from build123d import *

# Parameters (mm, degrees)
EXTRUDE_1_DEPTH     = 6
SKETCH_2_R          = 12
EXTRUDE_2_DEPTH     = 3
SKETCH_3_R          = 4.1
CUT_EXTRUDE_1_DEPTH = 64.788713735
CUT_EXTRUDE_2_DEPTH = 2
FILLET_1_R          = 0.5
SKETCH_5_R          = 12
SKETCH_5_R_2        = 4.1
EXTRUDE_3_DEPTH     = 6
FILLET_2_R          = 2


with BuildPart() as part:
    # Sketch 1 → Extrude 1 (new body)
    with BuildSketch(Plane(origin=(0, 0, 0), x_dir=(1, 0, 0), z_dir=(0, 1, 0))):
        with BuildLine():
            Line((-50, 9), (50, 9))
            ThreePointArc((50, 9), (59, 0), (50, -9))
            Line((50, -9), (-50, -9))
            ThreePointArc((-50, -9), (-59, 0), (-50, 9))
        make_face()
    extrude(amount=EXTRUDE_1_DEPTH)

    # Sketch 2 → Extrude 2 (add)
    with BuildSketch(Plane(origin=(0, 6, 0), x_dir=(1, 0, 0), z_dir=(0, 1, 0))):
        with Locations(Location((-50, 0, 0), (0, 0, 48.590377891))):
            Circle(SKETCH_2_R)
        with Locations(Location((50, 0, 0), (0, 0, 131.409622109))):
            Circle(SKETCH_2_R)
    extrude(amount=EXTRUDE_2_DEPTH)

    # Sketch 3 → Cut-Extrude 1 (cut, through all)
    with BuildSketch(Plane(origin=(0, 9, 0), x_dir=(1, 0, 0), z_dir=(0, 1, 0))):
        with Locations(Location((-50, 0, 0), (0, 0, 270))):
            Circle(SKETCH_3_R)
        with Locations(Location((50, 0, 0), (0, 0, 270))):
            Circle(SKETCH_3_R)
    extrude(amount=-CUT_EXTRUDE_1_DEPTH, mode=Mode.SUBTRACT)

    # Sketch 4 → Cut-Extrude 2 (cut)
    with BuildSketch(Plane(origin=(0, 6, 0), x_dir=(1, 0, 0), z_dir=(0, 1, 0))):
        with BuildLine():
            Line((-28, 4), (28, 4))
            ThreePointArc((28, 4), (32, 0), (28, -4))
            Line((28, -4), (-28, -4))
            ThreePointArc((-28, -4), (-32, 0), (-28, 4))
        make_face()
    extrude(amount=-CUT_EXTRUDE_2_DEPTH, mode=Mode.SUBTRACT)

    # Fillet 1
    fillet_1_edges = [part.edges().sort_by_distance(p)[0] for p in [
        (-57.937253933, 9, 9),
        (57.937253933, 9, 9),
    ]]
    fillet(fillet_1_edges, radius=FILLET_1_R)

    # Sketch 5 → Extrude 3 (add)
    # profile 1 of 2: a face of its own
    with BuildSketch(Plane.XZ):
        with Locations(Location((-50, 0, 0), (0, 0, 311.409622109))):
            Circle(SKETCH_5_R)
        with Locations(Location((-50, 0, 0), (0, 0, 90))):
            Circle(SKETCH_5_R_2, mode=Mode.SUBTRACT)
    # profile 2 of 2: a face of its own
    with BuildSketch(Plane.XZ):
        with Locations(Location((50, 0, 0), (0, 0, 228.590377891))):
            Circle(SKETCH_5_R)
        with Locations(Location((50, 0, 0), (0, 0, 90))):
            Circle(SKETCH_5_R_2, mode=Mode.SUBTRACT)
    extrude(amount=-EXTRUDE_3_DEPTH)

    # Fillet 2
    # the kernel refuses this fillet: 2 mm, written as the material it adds along each edge
    with BuildSketch(Plane(origin=(-42.062746067, 6, 9), x_dir=(-0.7681559640116129, 0, 0.6402627702384309), z_dir=(0, -1, 0))) as fillet_2_piece_1:
        with BuildLine():
            CenterArc((0.725148698, -1.999221978), FILLET_2_R, 91.598205704, 38.213210702)
            Line((-0.555376842, -0.46291005), (0, 0))
            ThreePointArc((0, 0), (0.334684015, -0.004668133), (0.669368029, 0))
        make_face()
    extrude(amount=6)
    with BuildSketch(Plane(origin=(-42.062746067, 0, -9), x_dir=(-0.7681559640131315, 0, -0.6402627702366088), z_dir=(0, 1, 0))) as fillet_2_piece_2:
        with BuildLine():
            CenterArc((0.725148698, -1.999221978), FILLET_2_R, 91.598205704, 38.213210702)
            Line((-0.555376842, -0.46291005), (0, 0))
            ThreePointArc((0, 0), (0.334684014, -0.004668133), (0.669368029, 0))
        make_face()
    extrude(amount=6)
    with BuildSketch(Plane(origin=(42.062746067, 6, 9), x_dir=(0.768155964011616, 0, 0.6402627702384273), z_dir=(0, -1, 0))) as fillet_2_piece_3:
        with BuildLine():
            CenterArc((0.725148698, 1.999221978), FILLET_2_R, 230.188583594, 38.213210702)
            Line((-0.555376842, 0.46291005), (0, 0))
            ThreePointArc((0, 0), (0.334684015, 0.004668133), (0.669368029, 0))
        make_face()
    extrude(amount=6)
    with BuildSketch(Plane(origin=(42.062746067, 0, -9), x_dir=(-1.0, 0, 5.1892707292062766e-11), z_dir=(0, 1, 0))) as fillet_2_piece_4:
        with BuildLine():
            CenterArc((0.723000105, -2), FILLET_2_R, 89.999999997, 38.213210702)
            ThreePointArc((-0.514179044, -0.428571429), (-0.25410069, -0.217871568), (0, 0))
            Line((0, 0), (0.723000105, 0))
        make_face()
    extrude(amount=6)


solid = part.part
For this review, take the finished solid that the model builds, in its own axes (mm). A direction names the side the tool comes from. Coordinates: 2 decimals unless noted, no trailing zeros. Loops run counter-clockwise (first coordinate to the right, second up) from the corner with the lowest first, then second, coordinate; pieces in that order, holes last. Notation, with made-up numbers: (7, 49.25) - (17, 49.25) arc R17 cw to (17, 63.25) - close; hole circle Ø4 at (60, 12.5). An arc over 180 degrees is marked (long way). Use a Markdown table: item, result. Add a question column.
Item 1: We need section D-D (x = -6.5). Give the boundary of the cut face in (y, z).
Item 2: We need section B-B (y = 2.25). Give the boundary of the cut face in (x, z).
Item 3: Insertion check: pin 1 Ø1.5 at (y, z) = (6, 5) entering from -X; pin 2 Ø3 at (x, y) = (45.5, 6.5) entering from -Z; pin 3 Ø2 at (y, z) = (4.5, -7) entering from -X. Each pin has a flat end and moves straight along its axis. Give the tip position at first contact, or say it passes through.
Item 4: For line 1 (X direction, y = 6.8, z = 0); line 2 (Z direction, x = 50, y = 4); line 3 (Z direction, x = -16, y = 5), list the stretches that pass through material, from the lowest coordinate up.
Item 5: We need section A-A (x = -50). Give the boundary of the cut face in (y, z), and give its area (3 significant figures).
Item 6: Tool access review of faces 1 (the face through (0, 5, -4)), 2 (the face through (-47, 9, -4)), 3 (the face through (1, 3, 9)): name each direction out of +Z, -Z, +X, -X, +Y, -Y from which nothing blocks a thin tool from reaching the whole face with its end or side.
Item 7: We need section C-C (z = 0). Give the boundary of the cut face in (x, y), and give its area (3 significant figures).
Item 8: Mouldability with a two-part tool opening along X and no side actions: class faces 4 (the face through (-1, 3, -9)), 5 (the face through (47, 9, -4)) as pulls with the +X half, pulls with the -X half, needs draft (parallel to the pull), parting line crosses it, or undercut.
Results list:
| question | item | result |
|---|---|---|
| 1 | outline | (0, -9) - (6, -9) - (6, -4) - (4, -4) - (4, 4) - (6, 4) - (6, 9) - (0, 9) - close |
| 2 | outline | (-42.58, -9.43) arc R2 cw to (-41.34, -9) - (41.34, -9) arc R2 cw to (42.58, -9.43) arc R12 ccw (long way) to (42.58, 9.43) arc R2 cw to (41.34, 9) - (-41.34, 9) arc R2 cw to (-42.58, 9.43) arc R12 ccw (long way) to start; hole circle Ø8.2 at (-50, 0); hole circle Ø8.2 at (50, 0) |
| 3 | pin 1 | stops at x = -61.22 |
| 3 | pin 2 | stops at z = -11.62 |
| 3 | pin 3 | stops at x = -60.39 |
| 4 | line 1 | x = -62 to -54.1, -45.9 to -38, 38 to 45.9, 54.1 to 62 |
| 4 | line 2 | z = -12 to -4.1, 4.1 to 12 |
| 4 | line 3 | z = -9 to -4, 4 to 9 |
| 5 | outline | (0, -12) - (8.5, -12) arc R0.5 ccw to (9, -11.5) - (9, -4.1) - (0, -4.1) - close; (0, 4.1) - (9, 4.1) - (9, 11.5) arc R0.5 ccw to (8.5, 12) - (0, 12) - close |
| 5 | area | 142 mm^2 |
| 6 | face 1 | +Y |
| 6 | face 2 | +Z, -Z, +X, -X, +Y |
| 6 | face 3 | +Z, +Y, -Y |
| 7 | outline | (-62, 0) - (-54.1, 0) - (-54.1, 9) - (-61.5, 9) arc R0.5 ccw to (-62, 8.5) - close; (-45.9, 0) - (45.9, 0) - (45.9, 9) - (38.5, 9) arc R0.5 ccw to (38, 8.5) - (38, 6) - (32, 6) - (32, 4) - (-32, 4) - (-32, 6) - (-38, 6) - (-38, 8.5) arc R0.5 ccw to (-38.5, 9) - (-45.9, 9) - close; (54.1, 0) - (62, 0) - (62, 8.5) arc R0.5 ccw to (61.5, 9) - (54.1, 9) - close |
| 7 | area | 612 mm^2 |
| 8 | face 4 | undercut |
| 8 | face 5 | needs draft |
